The figure shows three views and two pictorial views of one solid part (mm, origin at its lowest corner). Answer the questions. Coordinates: 2 decimals unless noted, no trailing zeros. Write each loop counter-clockwise with the first axis right and the second up, starting at its lowest first coordinate (ties: lowest second). Pieces come first, ordered by that corner, then holes. Notation, with made-up numbers: M 80.5,39 L 133.5,39 A31 ccw 133.5,68 Z; hole C 37,77 d5. An arc over 180 degrees is marked long. Write item = value, one per line.
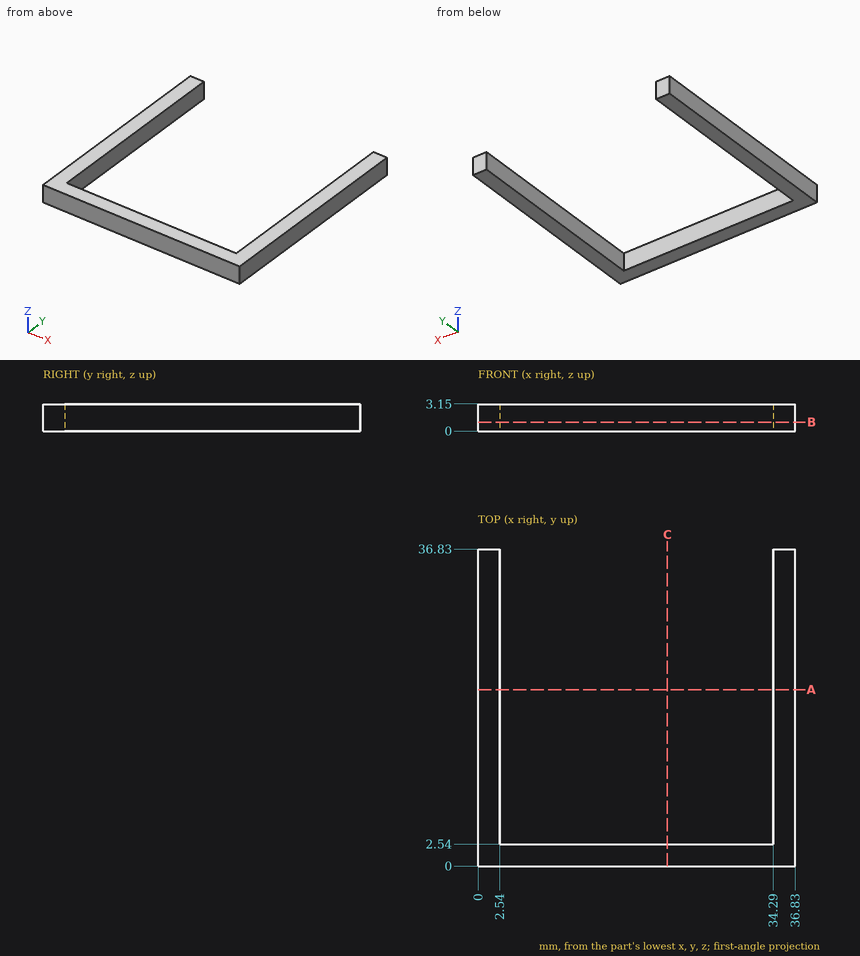
Item 1: Consider line 1 along X through (y, z) = (28.5, 1.8); line 2 along Y through (x, z) = (25.5, 0.4). Determine where each line is inside the solid, lowest interval first. Write a range as from..to.
Worked answers:
line_1 = 0..2.54, 34.29..36.83
line_2 = 0..2.54
Item 2: Find section B-B (z = 1.05). Determine the outline of the cut face in (x, y).
Worked answers:
outline = M 0,0 L 36.83,0 L 36.83,36.83 L 34.29,36.83 L 34.29,2.54 L 2.54,2.54 L 2.54,36.83 L 0,36.83 Z
Item 3: Find section A-A (y = 20.5). Determine the outline of the cut face in (x, z), and give its area (3 significant figures).
Worked answers:
outline = M 0,0 L 2.54,0 L 2.54,3.15 L 0,3.15 Z; M 34.29,0 L 36.83,0 L 36.83,3.15 L 34.29,3.15 Z
area = 16.0 mm²
Item 4: Find section C-C (x = 22). Determine the outline of the cut face in (y, z).
Worked answers:
outline = M 0,0 L 2.54,0 L 2.54,3.15 L 0,3.15 Z
